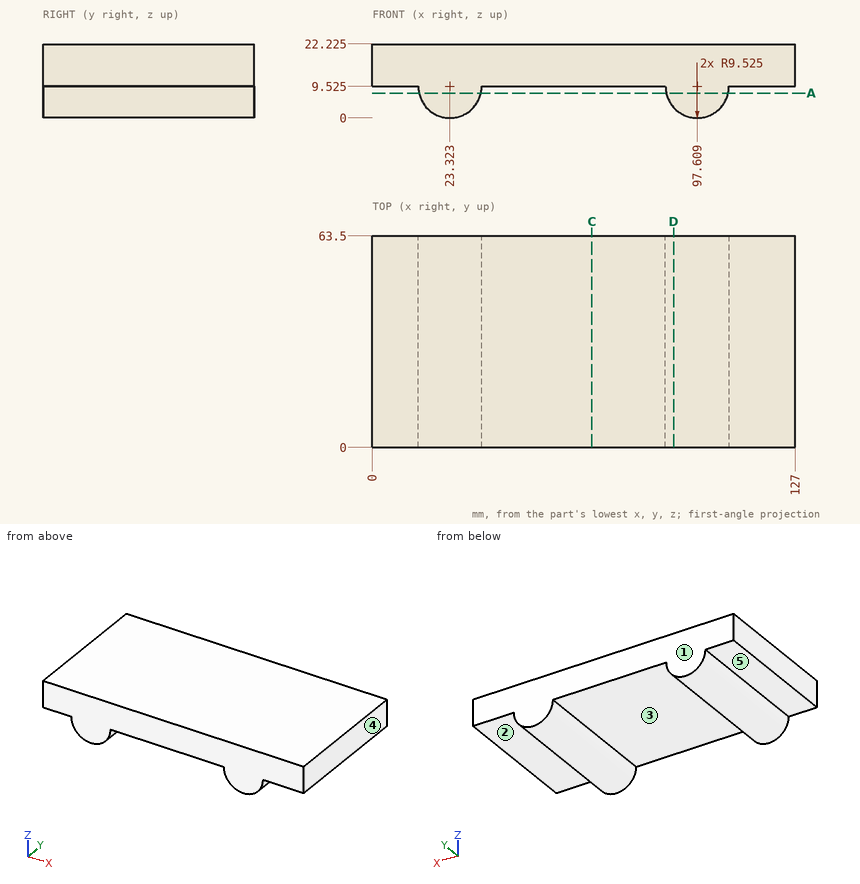
Source: three-view drawing plus pictorial views. Frame: mm from the lowest corner of the part. A direction names the side the tool comes from. Round coordinates to 2 decimals unless told otherwise and drop trailing zeros. Write each loop counter-clockwise with the first axis right and the second up, starting at its lowest first coordinate (ties: lowest second). Pieces come first, ordered by that corner, then holes. Notation, with made-up numbers: M 60,83 L 119,83 A9 ccw 119,94 Z; hole C 7.25,-40 d9. An arc over 180 degrees is marked long. Write each question's results on one line, items separated by ' | '.
Q1. Line query: line 1 along X through (y, z) = (39, 9.25); line 2 along Z through (x, y) = (84.5, 24) (3 decimals); line 3 along X through (y, z) = (3, 3). Output: solid intervals per line, ascending.
Results:
line 1: x = 13.8 to 32.84, 88.09 to 107.13 | line 2: z = 9.525 to 22.225 | line 3: x = 16.38 to 30.26, 90.67 to 104.55
Q2. Section query C-C (x = 66). Return loops of the section in (y, z) (3 decimals).
Results:
outline: M 0,9.525 L 63.5,9.525 L 63.5,22.225 L 0,22.225 Z
Q3. Section query A-A (z = 7.5). Return loops of the section in (x, y).
Results:
outline: M 14.02,0 L 32.63,0 L 32.63,63.5 L 14.02,63.5 Z; M 88.3,0 L 106.92,0 L 106.92,63.5 L 88.3,63.5 Z
Q4. Pin query (flat end, axial travel): P1, Ø11, axis at x = 10, y = 35.5, coming from the -Z side; P2, Ø4, axis at x = 41, y = 55.5, coming from the -Z side (3 decimals). Return the tip coordinate at first contact, or that it passes through.
Results:
P1: stops at z = 4.09 | P2: stops at z = 9.525
Q5. Draft query along X for the marked faces 3, 4 and 5. Return one class per face: released by +X, released by -X, zero draft, split by the parting line, or undercut.
Results:
face 3: undercut | face 4: released by +X | face 5: zero draft
Q6. Access query for the marked faces 1 and 2. Directions: +Z, -Z, +X, -X, +Y, -Y. A direction counts if a zero-diameter tool reaches every point of the face in a straight line with its end or side. Return the directions, or none.
Results:
face 1: +Z, -Z, +X, -X, +Y | face 2: -Z, +X, +Y, -Y
Q7. Section query D-D (x = 90.5). Return loops of the section in (y, z) (1 decimal).
Results:
outline: M 0,3.2 L 63.5,3.2 L 63.5,22.2 L 0,22.2 Z
